Design review of the part built by this model. Coordinates are the model's own, in mm. Face numbers are marked on the shaded views. A direction names the side the tool comes from. Give positions to 0.01 mm unless a question says otherwise; leave off trailing zeros. Order: outer loops, then holes, each group sorted by start corner. A loop starts at its lowest first (then second) coordinate and runs counter-clockwise, first axis right, second up. Notation, with made-up numbers: (86, 23) - (103, 23) arc R26 cw to (103, 59) - close; hole circle Ø5 at (-5, 24.5). An arc over 180 degrees is marked (long way). Write each question's results on one line, items separated by ' | '. Start each with the question number.
```python
from build123d import *

# Parameters (mm, degrees)
SKETCH1_W               = 16.9
SKETCH1_H               = 24
BOSS_EXTRUDE1_DEPTH     = 17
SKETCH2_W               = 12.7
SKETCH2_H               = 12.7
CUT_EXTRUDE1_DEPTH      = 23.458906919
SKETCH3_R               = 2.5
CUT_EXTRUDE2_DEPTH      = 31.600694437
BOSS_EXTRUDE2_DEPTH     = 12.7
EXTRUDE_3_DEPTH         = 4
EXTRUDE_4_DEPTH         = 4
SKETCH5_R               = 2.5
CUT_EXTRUDE3_DEPTH      = 30.49254143
SKETCH_4_W              = 3
SKETCH_4_H              = 16.9
CUT_EXTRUDE_1_DEPTH     = 32.937477984
SKETCH_5_W              = 12.7
SKETCH_5_H              = 1.5
CUT_EXTRUDE_2_DEPTH     = 30.320641194
CUT_EXTRUDE4_DEPTH      = 25.039394751
CUT_EXTRUDE4_DEPTH_BACK = 2
SKETCH_6_W              = 4
SKETCH_6_H              = 24
CUT_EXTRUDE_3_DEPTH     = 25.039394751
SKETCH_7_W              = 20.9
SKETCH_7_H              = 1.5
CUT_EXTRUDE_4_DEPTH     = 26.469442475
SKETCH_8_W              = 4
SKETCH_8_H              = 22.5
CUT_EXTRUDE_5_DEPTH     = 36.234819426
SKETCH_9_W              = 4
SKETCH_9_H              = 17
CUT_EXTRUDE_6_DEPTH     = 27.617663308
SKETCH_11_W             = 12.7
SKETCH_11_H             = 3.8
EXTRUDE_5_DEPTH         = 2
SKETCH_12_W             = 6
SKETCH_12_H             = 22.5
EXTRUDE_6_DEPTH         = 26.7
SKETCH_21_W             = 22.9
SKETCH_21_H             = 9.5
EXTRUDE_7_DEPTH         = 4
SKETCH_14_R             = 2.5
CUT_EXTRUDE_7_DEPTH     = 31.778239066
SKETCH_22_W             = 12
SKETCH_22_H             = 22.9
SKETCH_22_R             = 2.5
EXTRUDE_8_DEPTH         = 3


with BuildPart() as part:
    # Sketch1 → Boss-Extrude1 (new body)
    with BuildSketch(Plane(origin=(0, 0, 0), x_dir=(0, 0, -1), z_dir=(1, 0, 0))):
        Rectangle(SKETCH1_W, SKETCH1_H)
    extrude(amount=BOSS_EXTRUDE1_DEPTH)

    # Sketch2 → Cut-Extrude1 (cut, through all)
    with BuildSketch(Plane(origin=(17, 0, 0), x_dir=(0, 0, -1), z_dir=(1, 0, 0))):
        with Locations((2.1, -0.35)):
            Rectangle(SKETCH2_W, SKETCH2_H)
    extrude(amount=-CUT_EXTRUDE1_DEPTH, mode=Mode.SUBTRACT)

    # Sketch3 → Cut-Extrude2 (cut, through all)
    with BuildSketch(Plane(origin=(0, 12, 0), x_dir=(1, 0, 0), z_dir=(0, 1, 0))):
        with Locations(Location((7.63, 2.1, 0), (0, 0, 270))):
            Circle(SKETCH3_R)
    extrude(amount=-CUT_EXTRUDE2_DEPTH, mode=Mode.SUBTRACT)

    # Sketch4 → Boss-Extrude2 (add)
    with BuildSketch(Plane.ZY):
        Polygon((-8.45, 12), (-8.45, 6), (4.25, 6), (4.25, -12), (8.45, -12), (8.45, 12), align=None)
    extrude(amount=BOSS_EXTRUDE2_DEPTH)

    # 草图3 → 凸台-拉伸3 (add)
    with BuildSketch(Plane.ZY.offset(12.7)):
        Polygon((8.45, 12), (-7.55, 12), (8.45, -5), align=None)
    extrude(amount=EXTRUDE_3_DEPTH)

    # 草图1 → 凸台-拉伸4 (add)
    with BuildSketch(Plane(origin=(0, 0, -8.45), x_dir=(-1, 0, 0), z_dir=(0, 0, -1))):
        Polygon((12.7, 12), (0, 12), (0, 0.5), (-11.445354581, -12), (1.274949719, -12), (12.7, -12), align=None)
    extrude(amount=EXTRUDE_4_DEPTH)

    # Sketch5 → Cut-Extrude3 (cut, through all)
    with BuildSketch(Plane.XY.offset(8.45)):
        with Locations((-6.35, -1.63)):
            Circle(SKETCH5_R)
    extrude(amount=-CUT_EXTRUDE3_DEPTH, mode=Mode.SUBTRACT)

    # 草图4 → 切除-拉伸1 (cut, through all)
    with BuildSketch(Plane(origin=(0, 12, 0), x_dir=(1, 0, 0), z_dir=(0, 1, 0))):
        with Locations((15.5, 0)):
            Rectangle(SKETCH_4_W, SKETCH_4_H)
    extrude(amount=-CUT_EXTRUDE_1_DEPTH, mode=Mode.SUBTRACT)

    # 草图5 → 切除-拉伸2 (cut, through all)
    with BuildSketch(Plane.XY.offset(8.45)):
        with Locations((-6.35, -11.25)):
            Rectangle(SKETCH_5_W, SKETCH_5_H)
    extrude(amount=-CUT_EXTRUDE_2_DEPTH, mode=Mode.SUBTRACT)

    # Sketch7 → Cut-Extrude4 (cut, two sides: drawn at the far end of the back side and taken through both)
    with BuildSketch(Plane.ZY.offset(-CUT_EXTRUDE4_DEPTH_BACK)):
        Polygon((4.25, -6.7), (-8.45, -6.7), (-8.45, -10.5), (-12.45, -10.5), (-12.45, -12), (8.45, -12), (8.45, -10.5), (4.25, -10.5), align=None)
    extrude(amount=CUT_EXTRUDE4_DEPTH + CUT_EXTRUDE4_DEPTH_BACK, mode=Mode.SUBTRACT)

    # 草图6 → 切除-拉伸3 (cut, through all)
    with BuildSketch(Plane(origin=(0, 0, 0), x_dir=(0, 0, -1), z_dir=(1, 0, 0))):
        with Locations((10.45, 0)):
            Rectangle(SKETCH_6_W, SKETCH_6_H)
    extrude(amount=-CUT_EXTRUDE_3_DEPTH, mode=Mode.SUBTRACT)

    # 草图7 → 切除-拉伸4 (cut, through all)
    with BuildSketch(Plane.ZY.offset(-2)):
        with Locations((-2, -11.25)):
            Rectangle(SKETCH_7_W, SKETCH_7_H)
    extrude(amount=-CUT_EXTRUDE_4_DEPTH, mode=Mode.SUBTRACT)

    # 草图8 → 切除-拉伸5 (cut, through all)
    with BuildSketch(Plane(origin=(14, 0, 0), x_dir=(0, 0, -1), z_dir=(1, 0, 0))):
        with Locations((10.45, 0.75)):
            Rectangle(SKETCH_8_W, SKETCH_8_H)
    extrude(amount=-CUT_EXTRUDE_5_DEPTH, mode=Mode.SUBTRACT)

    # 草图9 → 切除-拉伸6 (cut, through all)
    with BuildSketch(Plane(origin=(0, 0, -8.45), x_dir=(-1, 0, 0), z_dir=(0, 0, -1))):
        with Locations((14.7, 3.5)):
            Rectangle(SKETCH_9_W, SKETCH_9_H)
    extrude(amount=-CUT_EXTRUDE_6_DEPTH, mode=Mode.SUBTRACT)

    # 草图11 → 凸台-拉伸5 (add)
    with BuildSketch(Plane.ZY.offset(-2)):
        with Locations((-2.1, -8.6)):
            Rectangle(SKETCH_11_W, SKETCH_11_H)
    extrude(amount=EXTRUDE_5_DEPTH)

    # 草图12 → 凸台-拉伸6 (add)
    with BuildSketch(Plane(origin=(14, 0, 0), x_dir=(0, 0, -1), z_dir=(1, 0, 0))):
        with Locations((11.45, 0.75)):
            Rectangle(SKETCH_12_W, SKETCH_12_H)
    extrude(amount=-EXTRUDE_6_DEPTH)

    # 草图21 → 凸台-拉伸7 (add)
    with BuildSketch(Plane.ZY.offset(12.7)):
        with Locations((-3, 7.25)):
            Rectangle(SKETCH_21_W, SKETCH_21_H)
    extrude(amount=EXTRUDE_7_DEPTH)

    # 草图14 → 切除-拉伸7 (cut, through all)
    with BuildSketch(Plane.XY.offset(8.45)):
        with Locations((-6.35, -1.63)):
            Circle(SKETCH_14_R)
    extrude(amount=-CUT_EXTRUDE_7_DEPTH, mode=Mode.SUBTRACT)

    # 草图22 → 凸台-拉伸8 (add)
    with BuildSketch(Plane.XZ.offset(10.5)):
        with Locations((8, -3)):
            Rectangle(SKETCH_22_W, SKETCH_22_H)
        with Locations(Location((7.63, -2.1, 0), (0, 0, 90))):
            Circle(SKETCH_22_R, mode=Mode.SUBTRACT)
    extrude(amount=EXTRUDE_8_DEPTH)


solid = part.part
```
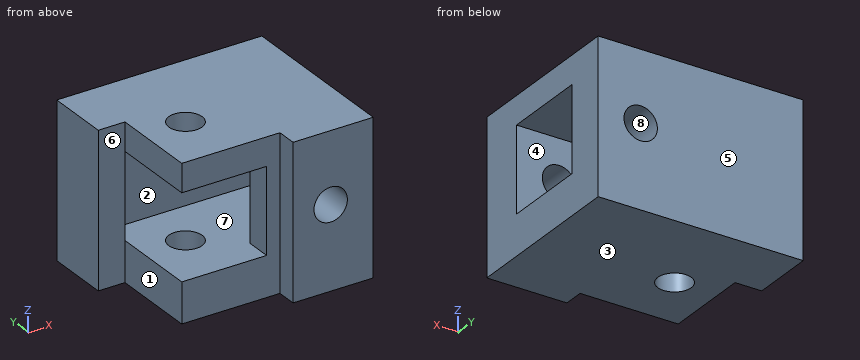
Q1. For line 1 (Y direction, x = 8, z = -6.25); line 2 (Z direction, x = -4.5, y = 1.5); line 3 (X direction, y = 10.45, z = -2.1), list the stretches that pass through material, from the lowest coordinate up. Write a range as [from, to].
Q2. Insertion check: pin 1 Ø3.5 at (y, z) = (-7, 7) entering from -X; pin 2 Ø4 at (y, z) = (-8, -4) entering from -X; pin 3 Ø4.5 at (x, y) = (-6.35, -1.63) entering from +Z; pin 4 Ø7.5 at (x, z) = (-5, 1) entering from -Y. Each pin has a flat end and moves straight along its axis. Give the tip position at first contact, or say it passes through.
Q3. Draft analysis for pull direction Y (two halves, no side actions). For the marked faces 5, 6, 7 and 8, state which applies: pulls with the +Y half, pulls with the -Y half, needs draft (parallel to the pull), parting line crosses it, or undercut.
Q4. Add section D-D (x = 0.5). Give the boundary of the cut face in (y, z), plus the area to 3 significant figures.
Q5. Machinability: for the marked faces 1, 2, 3 and 4, which of the approach directions +Z, -Z, +X, -X, +Y, -Y give a long, thin tool a straight path to every point of the face, cutting with its end or side? Answer none if there is none.
Q6. Add section C-C (z = -2.1). Give the boundary of the cut face in (x, y).
Q7. Add section B-B (y = -9.25). Give the boundary of the cut face in (x, z), plus the area to 3 significant figures.
Q8. Add section A-A (x = 7.63). Give the boundary of the cut face in (y, z), plus the area to 3 significant figures.
Verdict:
1) line 1: y = [-13.5, -6.7], [6, 12] | line 2: z = [-14.45, -8.45], [4.25, 8.45] | line 3: x = [-16.7, 5.13], [10.13, 14]
2) pin 1: stops at x = -12.7 | pin 2: stops at x = 0 | pin 3: passes through | pin 4: stops at y = -10.5
3) face 5: pulls with the +Y half | face 6: pulls with the -Y half | face 7: undercut | face 8: needs draft
4) outline: (-10.5, -14.45) - (12, -14.45) - (12, 8.45) - (-10.5, 8.45) - close; hole (-6.7, -8.45) - (6, -8.45) - (6, 4.25) - (-6.7, 4.25) - close | area: 354 mm2
5) face 1: +Z, -Z, -X, -Y | face 2: +X | face 3: -Z, +X, -X, +Y, -Y | face 4: +X, -X
6) outline: (-16.7, 2.5) - (-12.7, 2.5) - (-12.7, 6) - (5.13, 6) - (5.13, 12) - (-16.7, 12) - close; (0, -10.5) - (2, -10.5) - (2, -13.5) - (5.13, -13.5) - (5.13, -6.7) - (0, -6.7) - close; (10.13, -13.5) - (14, -13.5) - (14, -6.7) - (10.13, -6.7) - close; (10.13, 6) - (14, 6) - (14, 12) - (10.13, 12) - close
7) outline: (-12.7, -14.45) - (14, -14.45) - (14, 8.45) - (-12.7, 8.45) - (-12.7, 4.25) - (0, 4.25) - (0, -8.45) - (-12.7, -8.45) - close; hole circle Ø5 at (7.63, -2.1) | area: 431 mm2
8) outline: (-13.5, -14.45) - (12, -14.45) - (12, -4.6) - (6, -4.6) - (6, -8.45) - (-6.7, -8.45) - (-6.7, -4.6) - (-13.5, -4.6) - close; (-13.5, 0.4) - (-6.7, 0.4) - (-6.7, 4.25) - (6, 4.25) - (6, 0.4) - (12, 0.4) - (12, 8.45) - (-13.5, 8.45) - close | area: 359 mm2
